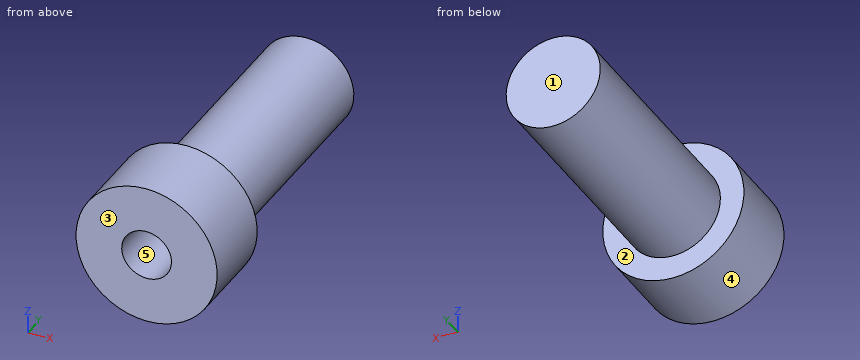
```python
from build123d import *

# Parameters (mm, degrees)
SKETCH_1_R          = 4.5
EXTRUDE_1_DEPTH     = 20
CUT_EXTRUDE_START   = -15
SKETCH_2_R          = 4.5
SKETCH_2_R_2        = 3
CUT_EXTRUDE_1_DEPTH = 15
SKETCH_3_R          = 1.5875
CUT_EXTRUDE_2_DEPTH = 15


with BuildPart() as part:
    # Эскиз1 → Бобышка-Вытянуть1 (new body)
    with BuildSketch(Plane(origin=(0, 0, 0), x_dir=(1, 0, 0), z_dir=(0, 1, 0))):
        with Locations(Location((0, 0, 0), (0, 0, 270))):
            Circle(SKETCH_1_R)
    extrude(amount=EXTRUDE_1_DEPTH)

    # Эскиз2 → Вырез-Вытянуть1 (cut)
    with BuildSketch(Plane(origin=(0, 20, 0), x_dir=(1, 0, 0), z_dir=(0, 1, 0)).offset(CUT_EXTRUDE_START)):
        with Locations(Location((0, 0, 0), (0, 0, 270))):
            Circle(SKETCH_2_R)
        with Locations(Location((0, 0, 0), (0, 0, 270))):
            Circle(SKETCH_2_R_2, mode=Mode.SUBTRACT)
    extrude(amount=CUT_EXTRUDE_1_DEPTH, mode=Mode.SUBTRACT)

    # Эскиз3 → Вырез-Вытянуть2 (cut)
    with BuildSketch(Plane.XZ):
        with Locations(Location((0, 0, 0), (0, 0, 270))):
            Circle(SKETCH_3_R)
    extrude(amount=-CUT_EXTRUDE_2_DEPTH, mode=Mode.SUBTRACT)


solid = part.part
```
Geometry: final body of the model. Coordinates: model frame, mm. Face numbers are marked on the shaded views. A direction names the side the tool comes from. Round coordinates to 2 decimals unless told otherwise and drop trailing zeros. Write each loop counter-clockwise with the first axis right and the second up, starting at its lowest first coordinate (ties: lowest second). Pieces come first, ordered by that corner, then holes. Notation, with made-up numbers: M 71.25,32 L 94.25,32 A9 cw 94.25,40 Z; hole C 2.25,37 d2. An arc over 180 degrees is marked long. Answer in a Markdown table with one row per item. Add a question column.
(1) Contact query for flat-ended pins moving along their axis: pin 1 (1.5 mm diameter, centred on y = 5, z = 1, fed in from -X); pin 2 (2.5 mm diameter, centred on x = 0, z = 0, fed in from -Y); pin 3 (3 mm diameter, centred on y = 12, z = -3, fed in from -X). Output: stop coordinate, or through.
(2) Ray query, L1, parallel to X at y = 7.5, z = 0; L2, parallel to Y at x = 1.25, z = 0.5; L3, parallel to Y at x = 2.5, z = 2.25. Return the intervals inside material, ascending.
(3) Cut plane D-D, the plane y = 16.25. Return the cut outline in (x, z).
(4) Cut plane B-B, the plane x = 0. Return the cut outline in (y, z), then the cut area to 3 significant figures.
(5) Reachability of the marked faces 1 and 2 from +Z, -Z, +X, -X, +Y, -Y: full face, straight path, thin tool, end or side. Return the list, or none.
(6) Cut plane C-C, the plane y = 12.5. Return the cut outline in (x, z) (1 decimal), then the cut area to 3 significant figures.
(7) Cut plane A-A, the plane z = 0. Return the cut outline in (x, y).
(8) Draft query along Z for the marked faces 3, 4 and 5. Return one class per face: pulls with the +Z half, pulls with the -Z half, needs draft (parallel to the pull), parting line crosses it, or undercut.
Established:
| question | item | result |
|---|---|---|
| 1 | pin 1 | x = -4.49 |
| 1 | pin 2 | y = 15 |
| 1 | pin 3 | x = -2.6 |
| 2 | L1 | -3 to -1.59, 1.59 to 3 |
| 2 | L2 | 15 to 20 |
| 2 | L3 | 0 to 5 |
| 3 | outline | C 0,0 d6 |
| 4 | outline | M 0,-4.5 L 5,-4.5 L 5,-3 L 20,-3 L 20,3 L 5,3 L 5,4.5 L 0,4.5 L 0,1.59 L 15,1.59 L 15,-1.59 L 0,-1.59 Z |
| 4 | area | 87.4 mm² |
| 5 | face 1 | +Z, -Z, +X, -X, +Y |
| 5 | face 2 | +Y |
| 6 | outline | C 0,0 d6; hole C 0,0 d3.2 |
| 6 | area | 20.4 mm² |
| 7 | outline | M -4.5,0 L -1.59,0 L -1.59,15 L 1.59,15 L 1.59,0 L 4.5,0 L 4.5,5 L 3,5 L 3,20 L -3,20 L -3,5 L -4.5,5 Z |
| 8 | face 3 | needs draft |
| 8 | face 4 | parting line crosses it |
| 8 | face 5 | undercut |
